CAD build for the part. Positions are in the model's coordinates, mm. A direction names the side the tool comes from. Give positions to 0.01 mm unless a question says otherwise; leave off trailing zeros. Loops run counter-clockwise (first coordinate to the right, second up) from the corner with the lowest first, then second, coordinate; pieces in that order, holes last.
```python
from build123d import *

# Parameters (mm, degrees)
SKETCH1_W           = 13.081
SKETCH1_H           = 8.128
BOSS_EXTRUDE1_DEPTH = 2.54
SKETCH2_R           = 0.5
CUT_EXTRUDE1_DEPTH  = 9.108380618
SKETCH3_R           = 1
CUT_EXTRUDE2_DEPTH  = 0.01


with BuildPart() as part:
    # Sketch1 → Boss-Extrude1 (new body)
    with BuildSketch(Plane(origin=(0, 0, 0), x_dir=(1, 0, 0), z_dir=(0, 1, 0))):
        Rectangle(SKETCH1_W, SKETCH1_H)
    extrude(amount=BOSS_EXTRUDE1_DEPTH)

    # Sketch2 → Cut-Extrude1 (cut, through all)
    with BuildSketch(Plane(origin=(0, 2.54, 0), x_dir=(1, 0, 0), z_dir=(0, 1, 0))):
        with Locations(Location((5.211297807, 2.563271845, 0), (0, 0, 270))):
            Circle(SKETCH2_R)
        with Locations(Location((5.211297807, 0.023271845, 0), (0, 0, 270))):
            Circle(SKETCH2_R)
        with Locations(Location((5.211297807, -2.516728155, 0), (0, 0, 270))):
            Circle(SKETCH2_R)
    extrude(amount=-CUT_EXTRUDE1_DEPTH, mode=Mode.SUBTRACT)

    # Sketch3 → Cut-Extrude2 (cut)
    with BuildSketch(Plane(origin=(0, 2.54, 0), x_dir=(1, 0, 0), z_dir=(0, 1, 0))):
        with Locations(Location((5.211297807, 2.563271845, 0), (0, 0, 270))):
            Circle(SKETCH3_R)
        with Locations(Location((5.211297807, 0.023271845, 0), (0, 0, 270))):
            Circle(SKETCH3_R)
        with Locations(Location((5.211297807, -2.516728155, 0), (0, 0, 270))):
            Circle(SKETCH3_R)
    extrude(amount=-CUT_EXTRUDE2_DEPTH, mode=Mode.SUBTRACT)


solid = part.part
```
1. Pull direction X, two halves, no side cores. Call faces 3 (the face through (-6.54, 1, 0)), 4 (the face through (5.707, 1.283, 2.452)), 5 (the face through (6.54, 1, 0)): released by +X, released by -X, zero draft, split by the parting line, or undercut.
Responses:
face 3: released by -X
face 4: undercut
face 5: released by +X
2. Tool access for faces 1 (the face through (6, 2.53, 0)), 2 (the face through (5.707, 1.283, -2.628)): list every direction of +Z, -Z, +X, -X, +Y, -Y with a clear straight run to the whole face (end or side of a thin tool).
Responses:
face 1: +Y
face 2: +Y, -Y
3. Drop a flat-ended pin along its axis: pin 1 (1 mm diameter, centred on x = 5.5, z = -2.5, fed in from +Y). Give the stop position or say it passes through.
Responses:
pin 1: stops at y = 2.53
4. Probe line 1 along X through (y, z) = (2.3, -2.25); line 2 along X through (y, z) = (1.85, -3); line 3 along Y through (x, z) = (4.5, -2). List the from-to ranges inside material, lowest first.
Responses:
line 1: x = -6.54 to 4.82, 5.6 to 6.54
line 2: x = -6.54 to 4.97, 5.45 to 6.54
line 3: y = 0 to 2.53
5. Saw through at B-B, the plane y = 0.8. List the corners of the cut face in (x, z).
Responses:
outline: (-6.54, -4.06) - (6.54, -4.06) - (6.54, 4.06) - (-6.54, 4.06) - close; hole circle Ø1 at (5.21, -2.56); hole circle Ø1 at (5.21, -0.02); hole circle Ø1 at (5.21, 2.52)
